Model file for the job. Use its own axes, mm. A direction names the side the tool comes from. Give positions to 0.01 mm unless a question says otherwise; leave off trailing zeros. Use a Markdown table: item, result.
from build123d import *

# Parameters (mm, degrees)
SKETCH_1_W      = 270
SKETCH_1_H      = 270
EXTRUDE_1_DEPTH = 20
FILLET_1_R      = 5
FILLET_2_R      = 8


with BuildPart() as part:
    # 草图1 → 凸台-拉伸1 (new body)
    with BuildSketch(Plane(origin=(0, 0, 0), x_dir=(1, 0, 0), z_dir=(0, 1, 0))):
        Rectangle(SKETCH_1_W, SKETCH_1_H)
    extrude(amount=EXTRUDE_1_DEPTH)

    # 草图2 → 旋转1 (revolve)
    with BuildSketch(Plane.XY):
        Polygon((0, 20), (125, 20), (110, 35), (75, 35), (71.498962309, 40), (31.498962309, 40), (21.498962309, 30), (0, 30), align=None)
    revolve(axis=Axis((0, 0, 0), (0, 1, 0)))

    # 圆角1
    fillet_1_edges = [part.edges().sort_by_distance(p)[0] for p in [
        (-125, 20, 0),
        (-75, 35, 0),
    ]]
    fillet(fillet_1_edges, radius=FILLET_1_R)

    # 圆角2
    fillet_2_edges = [part.edges().sort_by_distance(p)[0] for p in [
        (-71.498962309, 40, 0),
        (-110, 35, 0),
    ]]
    fillet(fillet_2_edges, radius=FILLET_2_R)


solid = part.part
(1) Pin check, flat tips, straight feed: P1, Ø5, axis at x = 66.5, y = 26, coming from the +Z side; P2, Ø12, axis at x = 18, z = 14, coming from the +Y side; P3, Ø1, axis at x = 61.5, y = 26, coming from the -Z side. Stop position of each tip, or through.
Computed:
| item | result |
|---|---|
| P1 | z = 102.1 |
| P2 | y = 37.3 |
| P3 | z = -102.53 |
(2) Drill centre lines: probe 1 along X at (y, z) = (33, -0.5); probe 2 along Y at (x, z) = (-2, 98); probe 3 along Z at (x, y) = (-3, 36.5). Where is each one in solid material? Low to high. Write a range as [from, to].
Computed:
| item | result |
|---|---|
| probe 1 | [-111.98, -24.49], [24.49, 111.98] |
| probe 2 | [0, 35] |
| probe 3 | [-73.97, -27.84], [27.84, 73.97] |
(3) 3-axis set-ups, long thin cutter, end or side, ignore diameter. For faces 1 (the flat face through (-2, 10, 135)), 2 (the flat face through (7, 35, 79)): which of +Z, -Z, +X, -X, +Y, -Y reach the whole face in a straight line?
Computed:
| item | result |
|---|---|
| face 1 | +Z, +X, -X, +Y, -Y |
| face 2 | +Y |
(4) Mould opens along X. For faces 3 (the flat face through (0, 30, 0)), 4 (the flat face through (135, 10, 2)), 5 (the flat face through (-135, 10, 2)), 6 (the flat face through (-1, 40, 32)) say: pulls with the +X half, pulls with the -X half, needs draft (parallel to the pull), parting line crosses it, or undercut.
Computed:
| item | result |
|---|---|
| face 3 | undercut |
| face 4 | pulls with the +X half |
| face 5 | pulls with the -X half |
| face 6 | needs draft |
